Geometry: final body of the model. Coordinates: model frame, mm. Give positions to 0.01 mm unless a question says otherwise; leave off trailing zeros. Order: outer loops, then holes, each group sorted by start corner. A loop starts at its lowest first (then second) coordinate and runs counter-clockwise, first axis right, second up. Notation, with made-up numbers: (-35, 20) -> (15, 20) arc R12 cw to (15, 38) -> close; hole circle Ø9 at (-15, -5.5). An arc over 180 degrees is marked (long way). Answer in a Markdown table with one row per item. Add a question column.
Q1. Contact query for flat-ended pins moving along their axis: P1, Ø7, axis at y = 8.5, z = 79, coming from the -X side; P2, Ø3, axis at x = -14.85, z = 214.85, coming from the -Y side; P3, Ø2.5, axis at y = 13, z = 0, coming from the +X side; P4, Ø3, axis at x = 1.5, y = 6, coming from the +Z side. Output: stop coordinate, or through.
Q2. Cut plane B-B on z = 131. Return the cut outline in (x, y).
Q3. Cut plane A-A on y = 4.75. Count the separate pieces of the cut face and the enclosed holes in it, and give its area (3 significant figures).
Q4. Line query: line 1 along X through (y, z) = (3.25, 15); line 2 along X through (y, z) = (9.5, -0.5); line 3 along X through (y, z) = (7.25, 160.5). Output: solid intervals per line, ascending. Write a range as from..to.
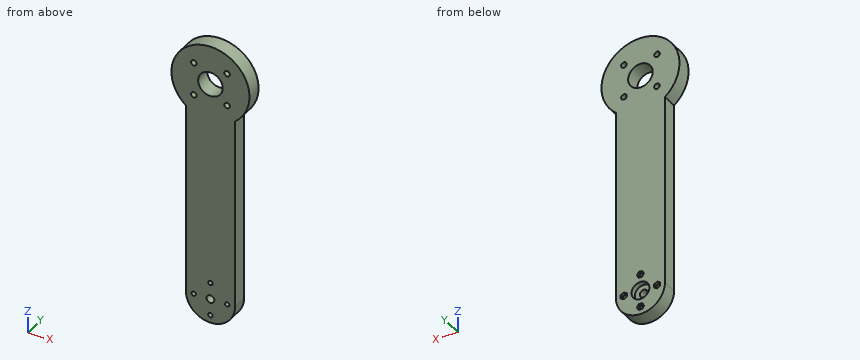
from build123d import *

# Parameters (mm, degrees)
BOSS_EXTRUDE1_DEPTH = 14
SKETCH2_R           = 8
CUT_EXTRUDE1_DEPTH  = 5
SKETCH3_R           = 3.5
CUT_EXTRUDE2_DEPTH  = 224.526284808
CUT_EXTRUDE9_DEPTH  = 2.4
SKETCH7_R           = 2
CUT_EXTRUDE10_DEPTH = 224.526284808
SKETCH8_R           = 35
BOSS_EXTRUDE2_DEPTH = 14
SKETCH9_R           = 2.5
SKETCH9_R_2         = 11
CUT_EXTRUDE11_DEPTH = 239.004201644


with BuildPart() as part:
    # Sketch1 → Boss-Extrude1 (new body)
    with BuildSketch(Plane(origin=(0, 0, 0), x_dir=(1, 0, 0), z_dir=(0, 1, 0))):
        with BuildLine():
            Line((-22, 0), (-22, -200))
            ThreePointArc((-22, -200), (0, -222), (22, -200))
            Line((22, -200), (22, 0))
            ThreePointArc((22, 0), (0, 22), (-22, 0))
        make_face()
    extrude(amount=BOSS_EXTRUDE1_DEPTH)

    # Sketch2 → Cut-Extrude1 (cut)
    with BuildSketch(Plane(origin=(0, 14, 0), x_dir=(1, 0, 0), z_dir=(0, 1, 0))):
        with Locations(Location((0, 0, 0), (0, 0, 270))):
            Circle(SKETCH2_R)
    extrude(amount=-CUT_EXTRUDE1_DEPTH, mode=Mode.SUBTRACT)

    # Sketch3 → Cut-Extrude2 (cut, through all)
    with BuildSketch(Plane(origin=(0, 14, 0), x_dir=(1, 0, 0), z_dir=(0, 1, 0))):
        with Locations(Location((0, 0, 0), (0, 0, 270))):
            Circle(SKETCH3_R)
    extrude(amount=-CUT_EXTRUDE2_DEPTH, mode=Mode.SUBTRACT)

    # Sketch4 → Cut-Extrude9 (cut)
    with BuildSketch(Plane(origin=(0, 14, 0), x_dir=(1, 0, 0), z_dir=(0, 1, 0))):
        Polygon((15, -3.175426481), (17.75, -1.58771324), (17.75, 1.58771324), (15, 3.175426481), (12.25, 1.58771324), (12.25, -1.58771324), align=None)
        Polygon((3.175426481, 15), (1.58771324, 17.75), (-1.58771324, 17.75), (-3.175426481, 15), (-1.58771324, 12.25), (1.58771324, 12.25), align=None)
        Polygon((-3.175426481, -15), (-1.58771324, -17.75), (1.58771324, -17.75), (3.175426481, -15), (1.58771324, -12.25), (-1.58771324, -12.25), align=None)
        Polygon((-15, 3.175426481), (-17.75, 1.58771324), (-17.75, -1.58771324), (-15, -3.175426481), (-12.25, -1.58771324), (-12.25, 1.58771324), align=None)
    extrude(amount=-CUT_EXTRUDE9_DEPTH, mode=Mode.SUBTRACT)

    # Sketch7 → Cut-Extrude10 (cut, through all)
    with BuildSketch(Plane(origin=(0, 14, 0), x_dir=(1, 0, 0), z_dir=(0, 1, 0))):
        with Locations(Location((0, 15, 0), (0, 0, 270))):
            Circle(SKETCH7_R)
        with Locations(Location((15, 0, 0), (0, 0, 270))):
            Circle(SKETCH7_R)
        with Locations(Location((0, -15, 0), (0, 0, 270))):
            Circle(SKETCH7_R)
        with Locations(Location((-15, 0, 0), (0, 0, 270))):
            Circle(SKETCH7_R)
    extrude(amount=-CUT_EXTRUDE10_DEPTH, mode=Mode.SUBTRACT)

    # Sketch8 → Boss-Extrude2 (add)
    with BuildSketch(Plane(origin=(0, 0, 0), x_dir=(1, 0, 0), z_dir=(0, 1, 0))):
        with Locations((0, -200)):
            Circle(SKETCH8_R)
    extrude(amount=BOSS_EXTRUDE2_DEPTH)

    # Sketch9 → Cut-Extrude11 (cut, through all)
    with BuildSketch(Plane(origin=(0, 14, 0), x_dir=(1, 0, 0), z_dir=(0, 1, 0))):
        with Locations(Location((-14.849242405, -185.150757595, 0), (0, 0, 270))):
            Circle(SKETCH9_R)
        with Locations(Location((14.849242405, -185.150757595, 0), (0, 0, 270))):
            Circle(SKETCH9_R)
        with Locations(Location((14.849242405, -214.849242405, 0), (0, 0, 270))):
            Circle(SKETCH9_R)
        with Locations(Location((-14.849242405, -214.849242405, 0), (0, 0, 270))):
            Circle(SKETCH9_R)
        with Locations(Location((0, -200, 0), (0, 0, 270))):
            Circle(SKETCH9_R_2)
    extrude(amount=-CUT_EXTRUDE11_DEPTH, mode=Mode.SUBTRACT)


solid = part.part
Completed:
| question | item | result |
|---|---|---|
| 1 | P1 | stops at x = -22 |
| 1 | P2 | passes through |
| 1 | P3 | stops at x = 22 |
| 1 | P4 | stops at z = 235 |
| 2 | outline | (-22, 0) -> (22, 0) -> (22, 14) -> (-22, 14) -> close |
| 3 | separate pieces | 1 |
| 3 | enclosed holes | 10 |
| 3 | area | 11,400 mm² |
| 4 | line 1 | x = -22..-2, 2..22 |
| 4 | line 2 | x = -21.99..-16.94, -13.06..-7.98, 7.98..13.06, 16.94..21.99 |
| 4 | line 3 | x = -22..22 |
